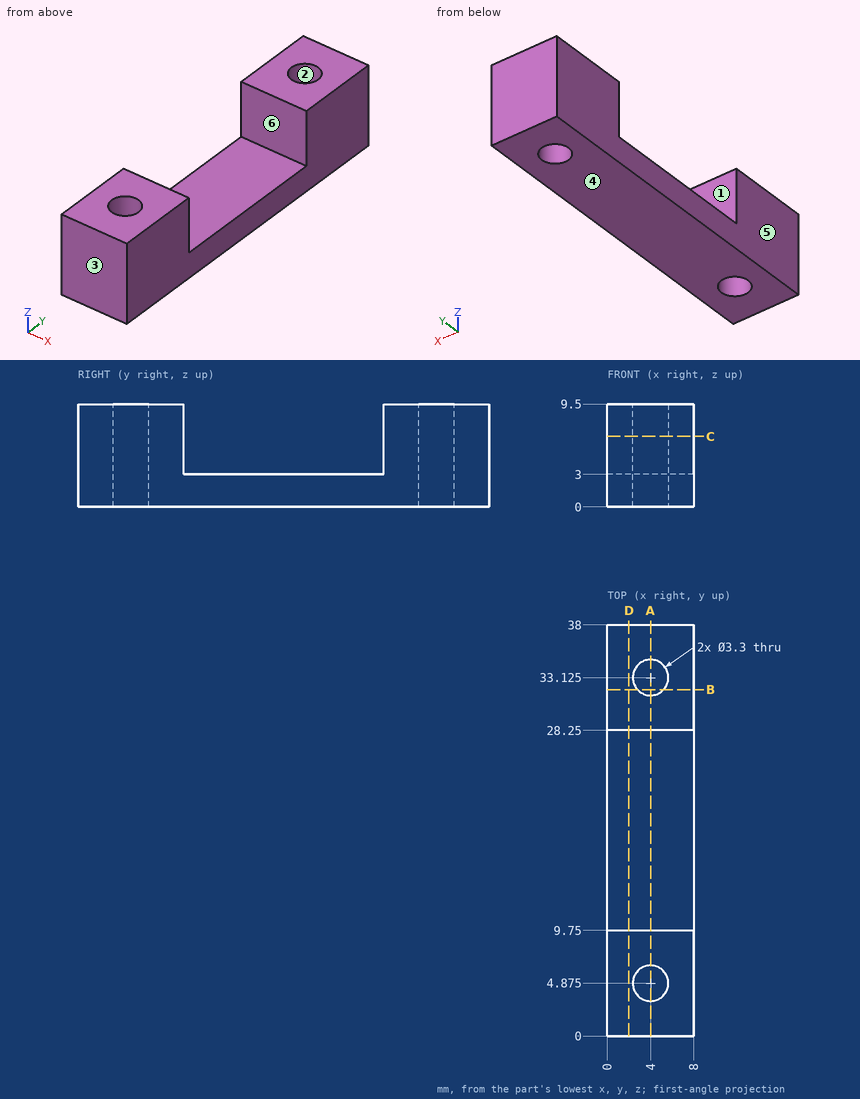
Source: three-view drawing plus pictorial views. Frame: mm from the lowest corner of the part. A direction names the side the tool comes from. Give positions to 0.01 mm unless a question says otherwise; leave off trailing zeros. Order: outer loops, then holes, each group sorted by start corner. A loop starts at its lowest first (then second) coordinate and runs counter-clockwise, first axis right, second up. Notation, with made-up numbers: (-12, 53) -> (28, 53) arc R18 ccw to (28, 58) -> close; hole circle Ø1 at (-29.5, 40). An arc over 180 degrees is marked (long way). Write each question's results on one line, items separated by ' | '. Start each with the question number.
Item 1: Set-up query: the marked faces 5 and 6. Return all of +Z, -Z, +X, -X, +Y, -Y with unobstructed straight access to the full face (end or side cutting, diameter ignored); none if empty.
Item 2: Cut plane B-B on y = 32. Return the cut outline in (x, z), then the cut area to 3 significant figures.
Item 3: Mould query, pull axis Y, two halves, no side actions, for the marked faces 1, 2, 3 and 4. Classes: pulls with the +Y half, pulls with the -Y half, needs draft (parallel to the pull), parting line crosses it, or undercut.
Item 4: Cut plane A-A on x = 4. Return the cut outline in (y, z) (3 decimals), then the cut area to 3 significant figures.
Item 5: Contact query for a flat-ended pin moving along its axis: P1, Ø4, axis at x = 3.5, y = 15.5, coming from the +Z side. Output: stop coordinate, or through.
Item 6: Cut plane D-D on x = 2. Return the cut outline in (y, z), then the cut area to 3 significant figures.
Item 7: Cut plane C-C on z = 6.5. Return the cut outline in (x, y) (3 decimals), then the cut area to 3 significant figures.
Item 8: Line query: line 1 (Y direction, x = 4, z = 7.25) (3 decimals); line 2 (Y direction, x = 4, z = 2.75) (3 decimals); line 3 (Y direction, x = 3, z = 4). Output: solid intervals per line, ascending.
Established:
1) face 5: +Z, -Z, -X, +Y, -Y | face 6: +Z, +X, -X
2) outline: (0, 0) -> (2.79, 0) -> (2.79, 9.5) -> (0, 9.5) -> close; (5.21, 0) -> (8, 0) -> (8, 9.5) -> (5.21, 9.5) -> close | area: 53.1 mm^2
3) face 1: undercut | face 2: undercut | face 3: pulls with the -Y half | face 4: needs draft
4) outline: (0, 0) -> (3.225, 0) -> (3.225, 9.5) -> (0, 9.5) -> close; (6.525, 0) -> (31.475, 0) -> (31.475, 9.5) -> (28.25, 9.5) -> (28.25, 3) -> (9.75, 3) -> (9.75, 9.5) -> (6.525, 9.5) -> close; (34.775, 0) -> (38, 0) -> (38, 9.5) -> (34.775, 9.5) -> close | area: 178 mm^2
5) P1: z = 3
6) outline: (0, 0) -> (38, 0) -> (38, 9.5) -> (28.25, 9.5) -> (28.25, 3) -> (9.75, 3) -> (9.75, 9.5) -> (0, 9.5) -> close | area: 241 mm^2
7) outline: (0, 0) -> (8, 0) -> (8, 9.75) -> (0, 9.75) -> close; (0, 28.25) -> (8, 28.25) -> (8, 38) -> (0, 38) -> close; hole circle Ø3.3 at (4, 4.875); hole circle Ø3.3 at (4, 33.125) | area: 139 mm^2
8) line 1: 0 to 3.225, 6.525 to 9.75, 28.25 to 31.475, 34.775 to 38 | line 2: 0 to 3.225, 6.525 to 31.475, 34.775 to 38 | line 3: 0 to 3.56, 6.19 to 9.75, 28.25 to 31.81, 34.44 to 38
